Verification items for the finished model (mm, model axes). Give positions to 0.01 mm unless a question says otherwise; leave off trailing zeros. Write each loop counter-clockwise with the first axis right and the second up, starting at its lowest first coordinate (ties: lowest second). Pieces come first, ordered by that corner, then holes.
from build123d import *

# Parameters (mm, degrees)
F0_R     = 10
F0_R_2   = 4
F0_R_3   = 7.5
F0_R_4   = 16
F1_DEPTH = 6


with BuildPart() as f1:
    # F0 (on Right) → F1 (new body)
    with BuildSketch(Plane.YZ):
        Polygon((-496, 0), (0, 0), (0, 600), (-200, 600), (-610, 200), (-610, 0), align=None)
        with Locations((-501, 25)):
            Circle(F0_R, mode=Mode.SUBTRACT)
        with Locations((-482, 16)):
            Circle(F0_R_2, mode=Mode.SUBTRACT)
        with Locations((-482, 67)):
            Circle(F0_R_2, mode=Mode.SUBTRACT)
        with Locations((-396, 17)):
            Circle(F0_R_3, mode=Mode.SUBTRACT)
        with Locations((-305, 22)):
            Circle(F0_R_4, mode=Mode.SUBTRACT)
        with Locations((-213, 17)):
            Circle(F0_R_3, mode=Mode.SUBTRACT)
        with Locations((-110, 24)):
            Circle(F0_R, mode=Mode.SUBTRACT)
        with Locations((-129, 66)):
            Circle(F0_R_2, mode=Mode.SUBTRACT)
        with Locations((-65, 18)):
            Circle(F0_R_2, mode=Mode.SUBTRACT)
    extrude(amount=F1_DEPTH)


solid = f1.part
Item 1: Sectioned sample at B-B on x = 2.5. State how many separate pieces and enclosed holes the cut face has, then the cut area to 3 significant figures.
Answer key:
separate pieces: 1
enclosed holes: 9
area: 282,000 mm2
Item 2: Sectioned sample at D-D on y = -213. Record the cut outline in (x, z).
Answer key:
outline: (0, 0) - (6, 0) - (6, 9.5) - (0, 9.5) - close; (0, 24.5) - (6, 24.5) - (6, 587.32) - (0, 587.32) - close
Item 3: Sectioned sample at A-A on y = -501. Record the cut outline in (x, z).
Answer key:
outline: (0, 0) - (6, 0) - (6, 15) - (0, 15) - close; (0, 35) - (6, 35) - (6, 306.34) - (0, 306.34) - close
Item 4: Sectioned sample at C-C on z = 326. Record the cut outline in (x, y), then the cut area to 3 significant figures.
Answer key:
outline: (0, -480.85) - (6, -480.85) - (6, 0) - (0, 0) - close
area: 2,890 mm2
Item 5: Scan lines: line 1 along Y through (x, z) = (5.3, 64); line 2 along Z through (x, y) = (4.35, -110); line 3 along Z through (x, y) = (2.9, -65). Record each from-to range of solid material in increasing order.
Answer key:
line 1: y = -610 to -484.65, -479.35 to -132.46, -125.54 to 0
line 2: z = 0 to 14, 34 to 600
line 3: z = 0 to 14, 22 to 600
Item 6: Release check for a two-part mould opening along Y. For faces 1 (the face through (0, -241, 238)), 2 (the face through (2.96, -389.07, 14.13)), 3 (the face through (2.96, -491.46, 28)), 4 (the face through (2.96, -402.13, 402.8)) record: released by +Y, released by -Y, zero draft, split by the parting line, or undercut.
Answer key:
face 1: zero draft
face 2: undercut
face 3: undercut
face 4: released by -Y
